```python
from build123d import *

# Parameters (mm, degrees)
SKETCH1_R               = 12.5
BOSS_EXTRUDE1_DEPTH     = 67
SKETCH14_R              = 16
BOSS_EXTRUDE2_DEPTH     = 29
SKETCH4_R               = 8.2804
CUT_EXTRUDE2_DEPTH      = 18
SKETCH8_OUTSIDE_W       = 50.17
SKETCH8_OUTSIDE_H       = 50.17
SKETCH8_OUTSIDE_R       = 12
CUT_EXTRUDE4_DEPTH      = 15
CHAMFER1_SIZE           = 1
SKETCH25_OUTSIDE_W      = 50.17
SKETCH25_OUTSIDE_H      = 50.17
SKETCH25_OUTSIDE_R      = 8
CUT_EXTRUDE7_DEPTH      = 20
CHAMFER2_SIZE           = 1
CUT_EXTRUDE8_DEPTH      = 71.717748833
CUT_EXTRUDE8_DEPTH_BACK = 71.717748833
SKETCH26_R              = 3


with BuildPart() as part:
    # Sketch1 → Boss-Extrude1 (new body)
    with BuildSketch(Plane(origin=(0, 0, 0), x_dir=(1, 0, 0), z_dir=(0, 1, 0))):
        with Locations(Location((0, 0, 0), (0, 0, 270))):
            Circle(SKETCH1_R)
    extrude(amount=BOSS_EXTRUDE1_DEPTH)

    # Sketch14 → Boss-Extrude2 (add)
    with BuildSketch(Plane(origin=(0, 67, 0), x_dir=(1, 0, 0), z_dir=(0, 1, 0))):
        with Locations(Location((0, 0, 0), (0, 0, 270))):
            Circle(SKETCH14_R)
    extrude(amount=-BOSS_EXTRUDE2_DEPTH)

    # Sketch4 → Cut-Extrude2 (cut)
    with BuildSketch(Plane(origin=(0, 67, 0), x_dir=(1, 0, 0), z_dir=(0, 1, 0))):
        with Locations(Location((0, 0, 0), (0, 0, 270))):
            Circle(SKETCH4_R)
    extrude(amount=-CUT_EXTRUDE2_DEPTH, mode=Mode.SUBTRACT)

    # Sketch8 outside → Cut-Extrude4 (cut)
    with BuildSketch(Plane(origin=(0, 67, 0), x_dir=(1, 0, 0), z_dir=(0, 1, 0))):
        Rectangle(SKETCH8_OUTSIDE_W, SKETCH8_OUTSIDE_H)
        with Locations(Location((0, 0, 0), (0, 0, 270))):
            Circle(SKETCH8_OUTSIDE_R, mode=Mode.SUBTRACT)
    extrude(amount=-CUT_EXTRUDE4_DEPTH, mode=Mode.SUBTRACT)

    # Chamfer1
    chamfer1_edges = [part.edges().sort_by_distance(p)[0] for p in [
        (0, 52, -16),
        (0, 38, -16),
    ]]
    chamfer(chamfer1_edges, length=CHAMFER1_SIZE)

    # Sketch25 outside → Cut-Extrude7 (cut)
    with BuildSketch(Plane.XZ):
        Rectangle(SKETCH25_OUTSIDE_W, SKETCH25_OUTSIDE_H)
        with Locations(Location((0, 0, 0), (0, 0, 270))):
            Circle(SKETCH25_OUTSIDE_R, mode=Mode.SUBTRACT)
    extrude(amount=-CUT_EXTRUDE7_DEPTH, mode=Mode.SUBTRACT)

    # Chamfer2
    chamfer2_edges = [part.edges().sort_by_distance(p)[0] for p in [
        (0, 67, -12),
        (0, 20, -12.5),
        (0, 0, 8),
    ]]
    chamfer(chamfer2_edges, length=CHAMFER2_SIZE)

    # Sketch26 → Cut-Extrude8 (cut, two sides: drawn at the far end of the back side and taken through both)
    with BuildSketch(Plane(origin=(0, 0, 0), x_dir=(0, 0, -1), z_dir=(1, 0, 0)).offset(-CUT_EXTRUDE8_DEPTH_BACK)):
        with Locations((0, 9.3)):
            Circle(SKETCH26_R)
    extrude(amount=CUT_EXTRUDE8_DEPTH + CUT_EXTRUDE8_DEPTH_BACK, mode=Mode.SUBTRACT)


solid = part.part
```
Work out the finished part from the listing and answer in its coordinate system (mm). A direction names the side the tool comes from. Round coordinates to 2 decimals unless told otherwise and drop trailing zeros. Loops run counter-clockwise (first coordinate to the right, second up) from the corner with the lowest first, then second, coordinate; pieces in that order, holes last. Notation, with made-up numbers: (58.25, 58) -> (91.25, 58) arc R13 cw to (91.25, 83) -> close; hole circle Ø4 at (33, 11). An arc over 180 degrees is marked (long way). Write each question's results on one line, items separated by ' | '. Start each with the question number.
1. For a pull along Z with two mould halves and no side action, classify faces 1 (the face through (0, 49, 0)), 2 (the face through (-15.62, 45.08, -3.47)), 3 (the face through (12.3, 38, -3.4)) as +Z half, -Z half, draft (parallel to the pull), parting line (faces both ways), or undercut.
2. Section D-D (y = 45) is taken. Determine the outline of the cut face in (x, z).
3. A tool of negligible diameter and unlimited length cuts with its end or side. For faces 4 (the face through (0, 0, 0)), 5 (the face through (-7, 52, -10)), 6 (the face through (3.755, 29.381, 11.923)), from which of +Z, -Z, +X, -X, +Y, -Y can it reach the whole face along a straight path? Write none if from no direction.
4. Section C-C (y = 60.5) is taken. Determine the outline of the cut face in (x, z).
5. Given pin 1 Ø5 at (x, z) = (-12, -4) entering from +Y; pin 2 Ø7 at (y, z) = (9.3, 0) entering from +X; pin 3 Ø1.5 at (x, y) = (-7.5, 45.5) entering from +Z; pin 4 Ø10 at (x, y) = (7, 18.5) entering from -Z, each flat-ended and moving along its own axis, determine where each tip first touches the part or whether it passes through.
6. Find the intervals of material crossed by probe 1 along X at (y, z) = (63.25, 0); probe 2 along Y at (x, z) = (8, 3.5); probe 3 along X at (y, z) = (43.5, 0), in increasing order. Write a range as from..to.
Evaluation:
1) face 1: undercut | face 2: parting line | face 3: draft
2) outline: circle Ø32 at (0, 0)
3) face 4: +Z, -Z, +X, -X, -Y | face 5: +Y | face 6: -Y
4) outline: circle Ø24 at (0, 0); hole circle Ø16.56 at (0, 0)
5) pin 1: stops at y = 67 | pin 2: stops at x = 8 | pin 3: stops at z = 14.51 | pin 4: stops at z = -12.21
6) probe 1: x = -12..-8.28, 8.28..12 | probe 2: y = 20..67 | probe 3: x = -16..16
